Can you work these out from the drawing? Everything is in mm from the part's minimum corner. A direction names the side the tool comes from. Round coordinates to 2 decimals unless told otherwise and drop trailing zeros. Write each loop counter-clockwise with the first axis right and the second up, starting at its lowest first coordinate (ties: lowest second). Pieces come first, ordered by that corner, then holes. Notation, with made-up numbers: (57, -28.5) -> (113, -28.5) arc R22 cw to (113, -9.5) -> close; hole circle Ø2 at (-7, 11). An arc over 180 degrees is marked (long way). Put each result on its own line as item: value. Start each with the question number.
1. Which directions (+Z, -Z, +X, -X, +Y, -Y) give clear straight access to the entire face, cutting with the end or side of a thin tool? Please do the marked faces 1 and 2.
2. I need wall thicknesses on probe 1 along Z at (x, y) = (5, 4.05); probe 2 along X at (y, z) = (3, 3); probe 3 along Y at (x, z) = (9, 5.25). Which ranges of each line are inside material? Lowest first, please. Write a range as from..to.
3. Suppose I cut it at C-C (x = 4). Please give me the cut outline in (y, z).
4. Suppose I cut it at A-A (z = 3). Please give me the cut outline in (x, y).
5. Suppose I cut it at B-B (y = 1.5). Please give me the cut outline in (x, z).
6. Suppose I cut it at D-D (z = 3.8). Please give me the cut outline in (x, y).
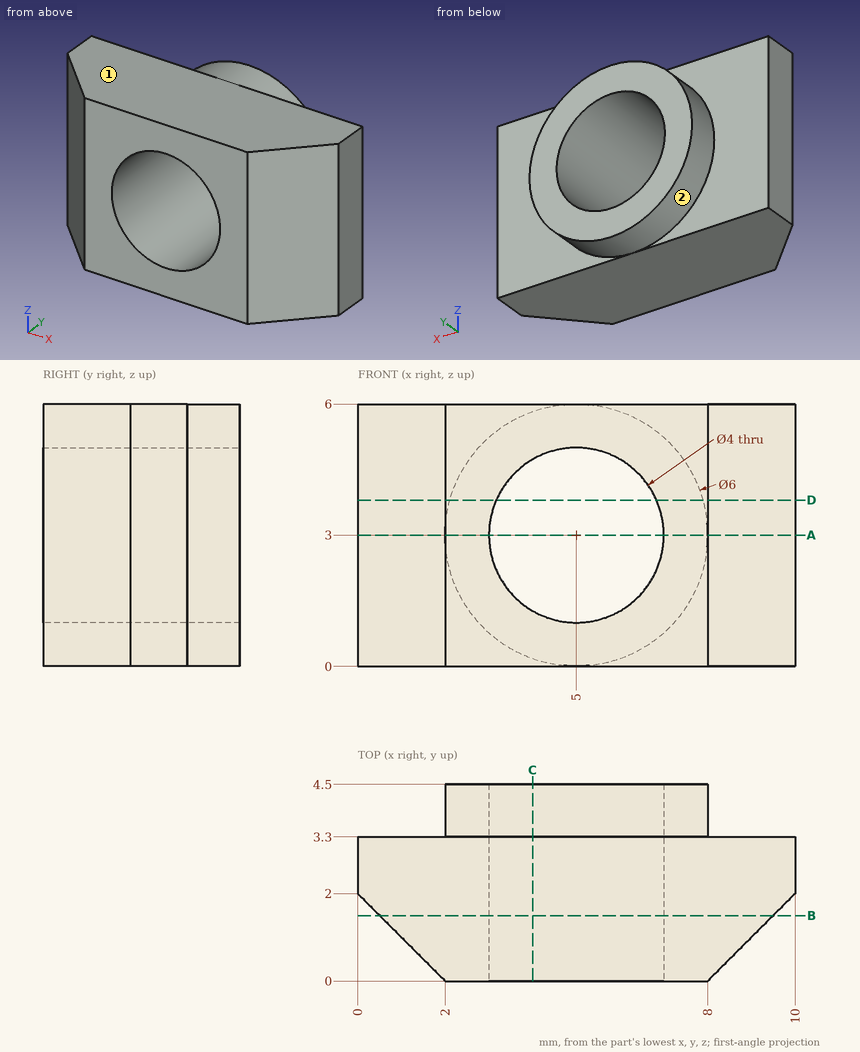
Verdict:
1. face 1: +Z, +X, -X, +Y, -Y
1. face 2: +Y
2. probe 1: z = 0..1, 5..6
2. probe 2: x = 0..3, 7..10
2. probe 3: y = 1..3.3
3. outline: (0, 0) -> (3.3, 0) -> (3.3, 0.17) -> (4.5, 0.17) -> (4.5, 1.27) -> (0, 1.27) -> close; (0, 4.73) -> (4.5, 4.73) -> (4.5, 5.83) -> (3.3, 5.83) -> (3.3, 6) -> (0, 6) -> close
4. outline: (0, 2) -> (2, 0) -> (3, 0) -> (3, 4.5) -> (2, 4.5) -> (2, 3.3) -> (0, 3.3) -> close; (7, 0) -> (8, 0) -> (10, 2) -> (10, 3.3) -> (8, 3.3) -> (8, 4.5) -> (7, 4.5) -> close
5. outline: (0.5, 0) -> (9.5, 0) -> (9.5, 6) -> (0.5, 6) -> close; hole circle Ø4 at (5, 3)
6. outline: (0, 2) -> (2, 0) -> (3.17, 0) -> (3.17, 4.5) -> (2.11, 4.5) -> (2.11, 3.3) -> (0, 3.3) -> close; (6.83, 0) -> (8, 0) -> (10, 2) -> (10, 3.3) -> (7.89, 3.3) -> (7.89, 4.5) -> (6.83, 4.5) -> close
